The listing builds one solid part. Answer for the finished solid, in the listing's coordinates (mm). A direction names the side the tool comes from. Give positions to 0.01 mm unless a question says otherwise; leave off trailing zeros. Write each loop counter-clockwise with the first axis right and the second up, starting at its lowest first coordinate (ties: lowest second). Pieces come first, ordered by that corner, then holes.
```python
from build123d import *

# Parameters (mm, degrees)
F1_DEPTH      = 9
F3_DEPTH      = 25
F4_DEPTH      = 3.2
F5_SIZE       = 0.2
F6_SIZE2      = 0.5358983849
F6_SIZE       = 2
F7_W          = 2.7641016151
F7_H          = 6
F8_DEPTH      = 6
F9_T4_DEPTH   = 37.1842967295
F9_T9_DEPTH   = 37.1842967295
F10_DEPTH     = 1
F11_DEPTH     = 1
F12_T4_DEPTH  = 5.2641016151
F12_T10_DEPTH = 5.2641016151
F12_T16_DEPTH = 5.2641016151
F12_T22_DEPTH = 5.2641016151
F12_T28_DEPTH = 5.2641016151
F12_T34_DEPTH = 5.2641016151
F12_T40_DEPTH = 5.2641016151
F12_T46_DEPTH = 5.2641016151
F12_T49_DEPTH = 12.2356354419


# Not quite as in the source:
# - a fillet or chamfer that OpenCascade refuses, or shapes differently, is made with other operations: its cross-section is extruded or revolved along the edge and cut away or added


with BuildPart() as f1:
    # F0 (on Top) → F1 (new body)
    with BuildSketch(Plane.XY):
        with BuildLine():
            Line((-34.4771644294, 42.6813552976), (-34.4771644294, 68.6813552976))
            ThreePointArc((-34.4771644294, 68.6813552976), (-35.0043722233, 69.9541475037), (-36.2771644294, 70.4813552976))
            Line((-36.2771644294, 70.4813552976), (-44.2771644294, 70.4813552976))
            ThreePointArc((-44.2771644294, 70.4813552976), (-45.5499566356, 69.9541475037), (-46.0771644294, 68.6813552976))
            Line((-46.0771644294, 68.6813552976), (-46.0771644294, 42.6813552976))
            ThreePointArc((-46.0771644294, 42.6813552976), (-45.5499566356, 41.4085630914), (-44.2771644294, 40.8813552976))
            Line((-44.2771644294, 40.8813552976), (-36.2771644294, 40.8813552976))
            ThreePointArc((-36.2771644294, 40.8813552976), (-35.0043722233, 41.4085630914), (-34.4771644294, 42.6813552976))
        make_face()
    extrude(amount=F1_DEPTH)

    # F2 (on face) → F3 (cut)
    with BuildSketch(Plane.XY.offset(9)):
        with BuildLine():
            ThreePointArc((-38.7771644294, 65.4813552976), (-39.2165042576, 66.5420154693), (-40.2771644294, 66.9813552976))
            ThreePointArc((-40.2771644294, 66.9813552976), (-41.3378246012, 64.4206951258), (-38.7771644294, 65.4813552976))
        make_face()
        with BuildLine():
            ThreePointArc((-38.7771644294, 45.8813552976), (-41.3378246012, 46.9420154693), (-40.2771644294, 44.3813552976))
            ThreePointArc((-40.2771644294, 44.3813552976), (-39.2165042576, 44.8206951258), (-38.7771644294, 45.8813552976))
        make_face()
    extrude(amount=-F3_DEPTH, mode=Mode.SUBTRACT)

    # F2 (on face) → F4 (cut)
    with BuildSketch(Plane.XY.offset(9)):
        with BuildLine():
            ThreePointArc((-37.4271644294, 65.4813552976), (-38.261910103, 67.4966096239), (-40.2771644294, 68.3313552976))
            ThreePointArc((-40.2771644294, 68.3313552976), (-42.2924187558, 63.4661009712), (-37.4271644294, 65.4813552976))
        make_face()
        with BuildLine():
            ThreePointArc((-38.7771644294, 65.4813552976), (-41.3378246012, 64.4206951258), (-40.2771644294, 66.9813552976))
            ThreePointArc((-40.2771644294, 66.9813552976), (-39.2165042576, 66.5420154693), (-38.7771644294, 65.4813552976))
        make_face(mode=Mode.SUBTRACT)
        with BuildLine():
            ThreePointArc((-37.4271644294, 45.8813552976), (-42.2924187558, 47.8966096239), (-40.2771644294, 43.0313552976))
            ThreePointArc((-40.2771644294, 43.0313552976), (-38.261910103, 43.8661009712), (-37.4271644294, 45.8813552976))
        make_face()
        with BuildLine():
            ThreePointArc((-38.7771644294, 45.8813552976), (-39.2165042576, 44.8206951258), (-40.2771644294, 44.3813552976))
            ThreePointArc((-40.2771644294, 44.3813552976), (-41.3378246012, 46.9420154693), (-38.7771644294, 45.8813552976))
        make_face(mode=Mode.SUBTRACT)
    extrude(amount=-F4_DEPTH, mode=Mode.SUBTRACT)

    # F5
    f5_edges = [f1.edges().sort_by_distance(p)[0] for p in [
        (-40.277164, 63.981355, 5.8),
        (-40.277164, 47.381355, 5.8),
        (-34.477164, 55.681355, 0),
        (-35.004372, 41.408563, 0),
        (-35.004372, 69.954148, 0),
        (-40.277164, 40.881355, 0),
        (-40.277164, 70.481355, 0),
        (-45.549957, 41.408563, 0),
        (-45.549957, 69.954148, 0),
        (-46.077164, 55.681355, 0),
        (-40.277164, 47.381355, 0),
        (-40.277164, 63.981355, 0),
        (-40.277164, 62.631355, 9),
        (-40.277164, 48.731355, 9),
    ]]
    chamfer(f5_edges, length=F5_SIZE)

    # F6
    f6_edges = [f1.edges().sort_by_distance(p)[0] for p in [
        (-34.477164, 55.681355, 9),
    ]]
    f6_side = f1.faces().sort_by_distance((-34.477164, 55.681355, 4.6))[0]
    chamfer(f6_edges, length=F6_SIZE, length2=F6_SIZE2, reference=f6_side)

    # F7 (on face) → F8 (join)
    with BuildSketch(Plane.XY.offset(9)):
        with Locations((-36.3951136219, 55.6813552976)):
            Rectangle(F7_W, F7_H)
        with Locations((-44.159215237, 55.6813552976)):
            Rectangle(F7_W, F7_H)
    extrude(amount=F8_DEPTH)

    # F9: chamfer of 1 x 6 on 2 edges, made by hand


with BuildPart() as f9_tool2:
    # F9_s3 → F9_t4 (new body)
    with BuildSketch(Plane.XZ.offset(-37.0892069328)):
        Polygon((-35.0130628143, 9), (-36.0130628143, 15), (-35.0130628143, 15), align=None)
    extrude(amount=-F9_T4_DEPTH)

    split(bisect_by=Plane(origin=(-30.4176323379, 0, -8.1503800206), x_dir=(0, 1, 0), z_dir=(0.9659258263, 0, 0.2588190451)), keep=Keep.TOP)


with BuildPart() as f1_1:
    add(f1.part)

    # F9_t1: cut F9_tool2
    add(f9_tool2.part, mode=Mode.SUBTRACT)


with BuildPart() as f9_tool7:
    # F9_s8 → F9_t9 (new body)
    with BuildSketch(Plane.XZ.offset(-74.2735036623)):
        Polygon((-45.5412660446, 9), (-44.5412660446, 15), (-45.5412660446, 15), align=None)
    extrude(amount=F9_T9_DEPTH)

    split(bisect_by=Plane(origin=(-44.7405796798, 0, 11.9882021941), x_dir=(0, 1, 0), z_dir=(-0.9659258263, 0, 0.2588190451)), keep=Keep.TOP)


with BuildPart() as f1_2:
    add(f1_1.part)

    # F9_t6: cut F9_tool7
    add(f9_tool7.part, mode=Mode.SUBTRACT)

    # F10 (add): faces of the model
    f10_faces = [f1_2.faces().sort_by_distance(p)[0] for p in [
        (-36.6267104431, 58.6813552976, 11.7791618553),
        (-43.9276184157, 58.6813552976, 11.7791618553),
    ]]
    extrude(f10_faces, amount=F10_DEPTH)

    # F11 (add): faces of the model
    f11_faces = [f1_2.faces().sort_by_distance(p)[0] for p in [
        (-43.9276184157, 52.6813552976, 11.7791618553),
        (-36.6267104431, 52.6813552976, 11.7791618553),
    ]]
    extrude(f11_faces, amount=F11_DEPTH)

    # F12: fillet of radius 1 on 6 edges, made by hand


with BuildPart() as f12_tool2:
    # F12_s3 → F12_t4 (new body)
    with BuildSketch(Plane.YZ.offset(-37.7771644294)):
        with BuildLine():
            ThreePointArc((50.6813552976, 9), (51.3884620788, 9.2928932188), (51.6813552976, 10))
            Line((51.6813552976, 10), (51.6813552976, 9))
            Line((51.6813552976, 9), (50.6813552976, 9))
        make_face()
    extrude(amount=F12_T4_DEPTH)

    split(bisect_by=Plane(origin=(-30.4176323379, 0, -8.1503800206), x_dir=(0, 1, 0), z_dir=(-0.9659258263, 0, -0.2588190451)), keep=Keep.TOP)

    split(bisect_by=Plane(origin=(-32.6073043599, 0, -5.4345507266), x_dir=(0, 1, 0), z_dir=(-0.9863939238, 0, -0.1643989873)), keep=Keep.TOP)


with BuildPart() as f1_3:
    add(f1_2.part)

    # F12_t1: union F12_tool2
    add(f12_tool2.part)


with BuildPart() as f12_tool8:
    # F12_s9 → F12_t10 (new body)
    with BuildSketch(Plane.YZ.offset(-37.7771644294)):
        with BuildLine():
            ThreePointArc((50.6813552976, 9), (51.3884620788, 9.2928932188), (51.6813552976, 10))
            Line((51.6813552976, 10), (51.6813552976, 9))
            Line((51.6813552976, 9), (50.6813552976, 9))
        make_face()
    extrude(amount=F12_T10_DEPTH)

    split(bisect_by=Plane(origin=(-30.4176323379, 0, -8.1503800206), x_dir=(0, 1, 0), z_dir=(0.9659258263, 0, 0.2588190451)), keep=Keep.TOP)

    split(bisect_by=Plane(origin=(-32.6073043599, 0, -5.4345507266), x_dir=(0, 1, 0), z_dir=(-0.9863939238, 0, -0.1643989873)), keep=Keep.TOP)


with BuildPart() as f1_4:
    add(f1_3.part)

    # F12_t7: union F12_tool8
    add(f12_tool8.part)


with BuildPart() as f12_tool14:
    # F12_s15 → F12_t16 (new body)
    with BuildSketch(Plane.YZ.offset(-48.0412660446)):
        with BuildLine():
            ThreePointArc((50.6813552976, 9), (51.3884620788, 9.2928932188), (51.6813552976, 10))
            Line((51.6813552976, 10), (51.6813552976, 9))
            Line((51.6813552976, 9), (50.6813552976, 9))
        make_face()
    extrude(amount=F12_T16_DEPTH)

    split(bisect_by=Plane(origin=(-44.7405796798, 0, 11.9882021941), x_dir=(0, 1, 0), z_dir=(-0.9659258263, 0, 0.2588190451)), keep=Keep.TOP)

    split(bisect_by=Plane(origin=(-45.7698804758, 0, 7.6283134126), x_dir=(0, 1, 0), z_dir=(0.9863939238, 0, -0.1643989873)), keep=Keep.TOP)


with BuildPart() as f1_5:
    add(f1_4.part)

    # F12_t13: union F12_tool14
    add(f12_tool14.part)


with BuildPart() as f12_tool20:
    # F12_s21 → F12_t22 (new body)
    with BuildSketch(Plane.YZ.offset(-48.0412660446)):
        with BuildLine():
            ThreePointArc((50.6813552976, 9), (51.3884620788, 9.2928932188), (51.6813552976, 10))
            Line((51.6813552976, 10), (51.6813552976, 9))
            Line((51.6813552976, 9), (50.6813552976, 9))
        make_face()
    extrude(amount=F12_T22_DEPTH)

    split(bisect_by=Plane(origin=(-44.7405796798, 0, 11.9882021941), x_dir=(0, 1, 0), z_dir=(0.9659258263, 0, -0.2588190451)), keep=Keep.TOP)

    split(bisect_by=Plane(origin=(-45.7698804758, 0, 7.6283134126), x_dir=(0, 1, 0), z_dir=(0.9863939238, 0, -0.1643989873)), keep=Keep.TOP)


with BuildPart() as f1_6:
    add(f1_5.part)

    # F12_t19: union F12_tool20
    add(f12_tool20.part)


with BuildPart() as f12_tool26:
    # F12_s27 → F12_t28 (new body)
    with BuildSketch(Plane.YZ.offset(-32.5130628143)):
        with BuildLine():
            ThreePointArc((60.6813552976, 9), (59.9742485164, 9.2928932188), (59.6813552976, 10))
            Line((59.6813552976, 10), (59.6813552976, 9))
            Line((59.6813552976, 9), (60.6813552976, 9))
        make_face()
    extrude(amount=-F12_T28_DEPTH)

    split(bisect_by=Plane(origin=(-30.4176323379, 0, -8.1503800206), x_dir=(0, 1, 0), z_dir=(0.9659258263, 0, 0.2588190451)), keep=Keep.TOP)

    split(bisect_by=Plane(origin=(-32.6073043599, 0, -5.4345507266), x_dir=(0, 1, 0), z_dir=(-0.9863939238, 0, -0.1643989873)), keep=Keep.TOP)


with BuildPart() as f1_7:
    add(f1_6.part)

    # F12_t25: union F12_tool26
    add(f12_tool26.part)


with BuildPart() as f12_tool32:
    # F12_s33 → F12_t34 (new body)
    with BuildSketch(Plane.YZ.offset(-32.5130628143)):
        with BuildLine():
            ThreePointArc((60.6813552976, 9), (59.9742485164, 9.2928932188), (59.6813552976, 10))
            Line((59.6813552976, 10), (59.6813552976, 9))
            Line((59.6813552976, 9), (60.6813552976, 9))
        make_face()
    extrude(amount=-F12_T34_DEPTH)

    split(bisect_by=Plane(origin=(-30.4176323379, 0, -8.1503800206), x_dir=(0, 1, 0), z_dir=(-0.9659258263, 0, -0.2588190451)), keep=Keep.TOP)

    split(bisect_by=Plane(origin=(-32.6073043599, 0, -5.4345507266), x_dir=(0, 1, 0), z_dir=(-0.9863939238, 0, -0.1643989873)), keep=Keep.TOP)


with BuildPart() as f1_8:
    add(f1_7.part)

    # F12_t31: union F12_tool32
    add(f12_tool32.part)


with BuildPart() as f12_tool38:
    # F12_s39 → F12_t40 (new body)
    with BuildSketch(Plane.YZ.offset(-42.7771644294)):
        with BuildLine():
            ThreePointArc((60.6813552976, 9), (59.9742485164, 9.2928932188), (59.6813552976, 10))
            Line((59.6813552976, 10), (59.6813552976, 9))
            Line((59.6813552976, 9), (60.6813552976, 9))
        make_face()
    extrude(amount=-F12_T40_DEPTH)

    split(bisect_by=Plane(origin=(-44.7405796798, 0, 11.9882021941), x_dir=(0, 1, 0), z_dir=(0.9659258263, 0, -0.2588190451)), keep=Keep.TOP)

    split(bisect_by=Plane(origin=(-45.7698804758, 0, 7.6283134126), x_dir=(0, 1, 0), z_dir=(0.9863939238, 0, -0.1643989873)), keep=Keep.TOP)


with BuildPart() as f1_9:
    add(f1_8.part)

    # F12_t37: union F12_tool38
    add(f12_tool38.part)


with BuildPart() as f12_tool44:
    # F12_s45 → F12_t46 (new body)
    with BuildSketch(Plane.YZ.offset(-42.7771644294)):
        with BuildLine():
            ThreePointArc((60.6813552976, 9), (59.9742485164, 9.2928932188), (59.6813552976, 10))
            Line((59.6813552976, 10), (59.6813552976, 9))
            Line((59.6813552976, 9), (60.6813552976, 9))
        make_face()
    extrude(amount=-F12_T46_DEPTH)

    split(bisect_by=Plane(origin=(-44.7405796798, 0, 11.9882021941), x_dir=(0, 1, 0), z_dir=(-0.9659258263, 0, 0.2588190451)), keep=Keep.TOP)

    split(bisect_by=Plane(origin=(-45.7698804758, 0, 7.6283134126), x_dir=(0, 1, 0), z_dir=(0.9863939238, 0, -0.1643989873)), keep=Keep.TOP)


with BuildPart() as f1_10:
    add(f1_9.part)

    # F12_t43: union F12_tool44
    add(f12_tool44.part)

    # F12_s50 → F12_t49 (cut)
    with BuildSketch(Plane.XZ.offset(-61.7991730185)):
        with BuildLine():
            ThreePointArc((-36.8601899027, 15), (-36.2138150066, 14.7630199825), (-35.8737959789, 14.1643989873))
            Line((-35.8737959789, 14.1643989873), (-36.0130628143, 15))
            Line((-36.0130628143, 15), (-36.8601899027, 15))
        make_face()
        with BuildLine():
            ThreePointArc((-44.68053288, 14.1643989873), (-44.3405138523, 14.7630199825), (-43.6941389562, 15))
            Line((-43.6941389562, 15), (-44.5412660446, 15))
            Line((-44.5412660446, 15), (-44.68053288, 14.1643989873))
        make_face()
    extrude(amount=F12_T49_DEPTH, mode=Mode.SUBTRACT)


solid = f1_10.part
```
Item 1: Which of the six approach directions +Z, -Z, +X, -X, +Y, -Y give full straight-line access (tool end or side, diameter ignored) to faces 1 (the face through (-42.777, 56, 12)), 2 (the face through (-40, 56, 9)), 3 (the face through (-35.185, 69.75, 8.014))?
Conclusion:
face 1: +Z, +Y, -Y
face 2: +Z
face 3: +Z, +X, +Y
Item 2: A cutting plane is placed at D-D, the plane z = 4.25. Give the vertices of the cut face in (x, y).
Conclusion:
outline: (-46.08, 42.68) arc R1.8 ccw to (-44.28, 40.88) - (-36.28, 40.88) arc R1.8 ccw to (-34.48, 42.68) - (-34.48, 68.68) arc R1.8 ccw to (-36.28, 70.48) - (-44.28, 70.48) arc R1.8 ccw to (-46.08, 68.68) - close; hole circle Ø3 at (-40.28, 45.88); hole circle Ø3 at (-40.28, 65.48)
Item 3: A cutting plane is placed at C-C, the plane z = 13. Give the vertices of the cut face in (x, y), plus the area to 3 significant figures.
Conclusion:
outline: (-44.87, 51.68) - (-42.78, 51.68) - (-42.78, 59.68) - (-44.87, 59.68) - close; (-37.78, 51.68) - (-35.68, 51.68) - (-35.68, 59.68) - (-37.78, 59.68) - close
area: 33.6 mm2
Item 4: A cutting plane is placed at A-A, the plane z = 6.5. Give the vertices of the cut face in (x, y), plus the area to 3 significant figures.
Conclusion:
outline: (-46.08, 42.68) arc R1.8 ccw to (-44.28, 40.88) - (-36.28, 40.88) arc R1.8 ccw to (-34.48, 42.68) - (-34.48, 68.68) arc R1.8 ccw to (-36.28, 70.48) - (-44.28, 70.48) arc R1.8 ccw to (-46.08, 68.68) - close; hole circle Ø5.7 at (-40.28, 45.88); hole circle Ø5.7 at (-40.28, 65.48)
area: 290 mm2
Item 5: A cutting plane is placed at B-B, the plane y = 57.5. Give the vertices of the cut face in (x, z), plus the area to 3 significant figures.
Conclusion:
outline: (-46.08, 0.2) - (-45.88, 0) - (-34.68, 0) - (-34.48, 0.2) - (-34.48, 7) - (-35.01, 9) - (-35.87, 14.16) arc R1 ccw to (-36.86, 15) - (-37.78, 15) - (-37.78, 9) - (-42.78, 9) - (-42.78, 15) - (-43.69, 15) arc R1 ccw to (-44.68, 14.16) - (-45.54, 9) - (-46.08, 7) - close
area: 130 mm2
Item 6: Determine the mould class of faces 4 (the face through (-36.376, 59.982, 9.285)), 5 (the face through (-39, 64, 5.8)), 6 (the face through (-45.56, 41.42, 3.55)), 7 (the face through (-34.99, 69.94, 3.55)) for opening direction X: pulls with the +X half, pulls with the -X half, needs draft (parallel to the pull), parting line crosses it, or undercut.
Conclusion:
face 4: needs draft
face 5: undercut
face 6: pulls with the -X half
face 7: pulls with the +X half
Item 7: Each of these flat-tipped pins is pushed along its axis until it touches: P1, Ø0.8, axis at x = -44.5, z = 13, coming from the -Y side; P2, Ø4, axis at x = -40.28, y = 45.88, coming from the +Z side; P3, Ø1.8, axis at y = 56, z = 12.5, coming from the +X side. Where does it stop, or does it pass through?
Conclusion:
P1: stops at y = 51.68
P2: stops at z = 5.8
P3: stops at x = -35.45
Item 8: Consider probe 1 along Z at (x, y) = (-41.25, 54.5); probe 2 along X at (y, z) = (46, 1); probe 3 along X at (y, z) = (45, 8.75). Determine where each line is inside the solid, lowest interval first.
Conclusion:
probe 1: z = 0 to 9
probe 2: x = -46.08 to -41.77, -38.78 to -34.48
probe 3: x = -45.61 to -42.99, -37.57 to -34.95
